```python
from build123d import *

# Parameters (mm, degrees)
SKETCH1_R           = 4.5
BOSS_EXTRUDE1_DEPTH = 10
SKETCH2_W           = 18
SKETCH2_H           = 14
BOSS_EXTRUDE2_DEPTH = 50
SKETCH4_R           = 1.5
SKETCH4_W           = 13
SKETCH4_H           = 9.5
BOSS_EXTRUDE3_DEPTH = 10
LOFT2_START         = -9
LOFT2_DEPTH         = 18
FILLET4_R           = 3


# Read off the part's stored shape, not the designer's step: Loft2
with BuildPart() as part:
    # Sketch1 → Boss-Extrude1 (new body)
    with BuildSketch(Plane(origin=(0, 0, 0), x_dir=(1, 0, 0), z_dir=(0, 1, 0))):
        with BuildLine():
            Line((-32, 10), (32, 10))
            ThreePointArc((32, 10), (42, 0), (32, -10))
            Line((32, -10), (-32, -10))
            ThreePointArc((-32, -10), (-42, 0), (-32, 10))
        make_face()
        with Locations(Location((-32, 0, 0), (0, 0, 270))):
            Circle(SKETCH1_R, mode=Mode.SUBTRACT)
        with Locations(Location((32, 0, 0), (0, 0, 270))):
            Circle(SKETCH1_R, mode=Mode.SUBTRACT)
    extrude(amount=BOSS_EXTRUDE1_DEPTH)

    # Sketch2 → Boss-Extrude2 (add)
    with BuildSketch(Plane(origin=(0, 10, 0), x_dir=(1, 0, 0), z_dir=(0, 1, 0))):
        with Locations((0, -3)):
            Rectangle(SKETCH2_W, SKETCH2_H)
    extrude(amount=BOSS_EXTRUDE2_DEPTH)



with BuildPart() as body_2:
    # Sketch4 → Boss-Extrude3 (new body)
    with BuildSketch(Plane(origin=(0, 60, 0), x_dir=(1, 0, 0), z_dir=(0, 1, 0))):
        Polygon((-25, 10), (-25, 27), (0, 27), (25, 27), (25, 10), (9, 4), (-9, 4), align=None)
        with Locations(Location((-21.5, 18.5, 0), (0, 0, 270))):
            Circle(SKETCH4_R, mode=Mode.SUBTRACT)
        with Locations(Location((-3.5, 18.5, 0), (0, 0, 270))):
            Circle(SKETCH4_R, mode=Mode.SUBTRACT)
        with Locations(Location((3.5, 18.5, 0), (0, 0, 90))):
            Circle(SKETCH4_R, mode=Mode.SUBTRACT)
        with Locations(Location((21.5, 18.5, 0), (0, 0, 90))):
            Circle(SKETCH4_R, mode=Mode.SUBTRACT)
        with Locations((-12.5, 18.5)):
            Rectangle(SKETCH4_W, SKETCH4_H, mode=Mode.SUBTRACT)
        with Locations((12.5, 18.5)):
            Rectangle(SKETCH4_W, SKETCH4_H, mode=Mode.SUBTRACT)
    extrude(amount=BOSS_EXTRUDE3_DEPTH)


with BuildPart() as part_1:
    add(part.part)

    add(body_2.part)  # Loft2 merges body 2
    # Loft2 outline → Loft2 (add)
    with BuildSketch(Plane.YZ.offset(LOFT2_START)):
        Polygon((60, -4), (70, -4), (60, 10), align=None)
    extrude(amount=LOFT2_DEPTH)

    # Fillet4
    fillet4_edges = [part_1.edges().sort_by_distance(p)[0] for p in [
        (0, 10, -10),
        (-42, 10, 0),
        (42, 10, 0),
        (9, 35, 10),
        (9, 10, 3),
        (-9, 10, 3),
        (20.5, 10, 10),
        (-20.5, 10, 10),
        (25, 65, -10),
        (25, 65, -27),
        (-25, 65, -27),
        (-9, 35, 10),
    ]]
    fillet(fillet4_edges, radius=FILLET4_R)


solid = part_1.part
```
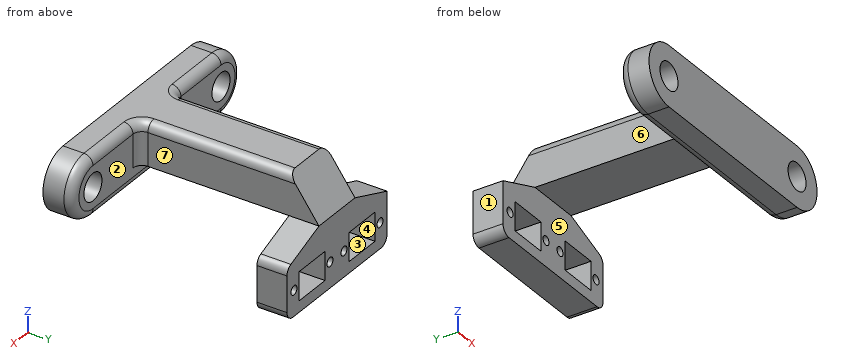
CAD build for the part. Positions are in the model's coordinates, mm. Face numbers are marked on the shaded views. A direction names the side the tool comes from. Coordinates: 2 decimals unless noted, no trailing zeros. Order: outer loops, then holes, each group sorted by start corner. A loop starts at its lowest first (then second) coordinate and runs counter-clockwise, first axis right, second up. Notation, with made-up numbers: (20, 60.5) - (60, 60.5) arc R24 cw to (60, 95.5) - close; hole circle Ø11 at (55.5, 27.5). An arc over 180 degrees is marked (long way). Answer in a Markdown table with one row per item.
1. Flat gauge pins, fed straight in: P1, Ø2, axis at x = -25.5, z = -21, coming from the -Y side; P2, Ø12, axis at y = 56, z = 5, coming from the +X side; P3, Ø8, axis at y = 66, z = -19, coming from the -X side; P4, Ø1.5, axis at x = 8.5, z = -19, coming from the -Y side. Where does each tip first touch, or does it go through?
Answer:
| item | result |
|---|---|
| P1 | y = 60 |
| P2 | x = 9 |
| P3 | x = -25 |
| P4 | through |
2. Pull direction X, two halves, no side cores. Call the marked faces 1, 2 and 3: +X half, -X half, draft (parallel to the pull), parting line (faces both ways), or undercut.
Answer:
| item | result |
|---|---|
| face 1 | -X half |
| face 2 | draft |
| face 3 | undercut |
3. 3-axis set-ups, long thin cutter, end or side, ignore diameter. For the marked faces 4, 5, 6 and 7: which of +Z, -Z, +X, -X, +Y, -Y reach the whole face in a straight line?
Answer:
| item | result |
|---|---|
| face 4 | +Y, -Y |
| face 5 | -Z, +X, -X |
| face 6 | +Z, -X, +Y |
| face 7 | +Z, +X, +Y |
4. Slice it at C-C, the plane y = 6. List the corners of the cut face in (x, z), then the cut area to 3 significant figures.
Answer:
| item | result |
|---|---|
| outline | (-32, -10) - (32, -10) arc R10 ccw to (32, 10) - (-32, 10) arc R10 ccw to start; hole circle Ø9 at (-32, 0); hole circle Ø9 at (32, 0) |
| area | 1,470 mm² |
5. Drill centre lines: L1, parallel to X at y = 3.25, z = 0; L2, parallel to Y at x = -27, z = -2; L3, parallel to X at y = 64, z = -3. Where is each one in solid material? Low to high. Write a range as from..to.
Answer:
| item | result |
|---|---|
| L1 | -42..-36.5, -27.5..27.5, 36.5..42 |
| L2 | 0..10 |
| L3 | -9..9 |
6. Slice it at D-D, the plane x = 13.5. List the corners of the cut face in (y, z).
Answer:
| item | result |
|---|---|
| outline | (0, -10) - (7, -10) arc R3 ccw to (10, -7) - (10, 7) arc R3 ccw to (7, 10) - (0, 10) - close; (60, -27) - (70, -27) - (70, -23.25) - (60, -23.25) - close; (60, -13.75) - (70, -13.75) - (70, -5.69) - (60, -5.69) - close |
7. Slice it at B-B, the plane x = 3.5. List the corners of the cut face in (y, z).
Answer:
| item | result |
|---|---|
| outline | (0, -10) - (7, -10) arc R3 ccw to (10, -7) - (10, -4) - (60, -4) - (60, -17) - (70, -17) - (70, -4) - (60, 10) - (0, 10) - close; (60, -27) - (70, -27) - (70, -20) - (60, -20) - close |
8. Slice it at A-A, the plane z = -18.5. List the corners of the cut face in (x, y), then the cut area to 3 significant figures.
Answer:
| item | result |
|---|---|
| outline | (-25, 60) - (-23, 60) - (-23, 70) - (-25, 70) - close; (-20, 60) - (-19, 60) - (-19, 70) - (-20, 70) - close; (-6, 60) - (-5, 60) - (-5, 70) - (-6, 70) - close; (-2, 60) - (2, 60) - (2, 70) - (-2, 70) - close; (5, 60) - (6, 60) - (6, 70) - (5, 70) - close; (19, 60) - (20, 60) - (20, 70) - (19, 70) - close; (23, 60) - (25, 60) - (25, 70) - (23, 70) - close |
| area | 120 mm² |
